Geometry check sheet. Reference: drawing and pictorial views, mm from the part's lowest x, y, z. Coordinates: 2 decimals unless noted, no trailing zeros. Write each loop counter-clockwise with the first axis right and the second up, starting at its lowest first coordinate (ties: lowest second). Pieces come first, ordered by that corner, then holes. Notation, with made-up numbers: (8, 16) -> (52, 16) arc R23 cw to (52, 45) -> close; hole circle Ø9 at (76, 38.25). An arc over 180 degrees is marked (long way). Use a Markdown table: item, result. Add a question column.
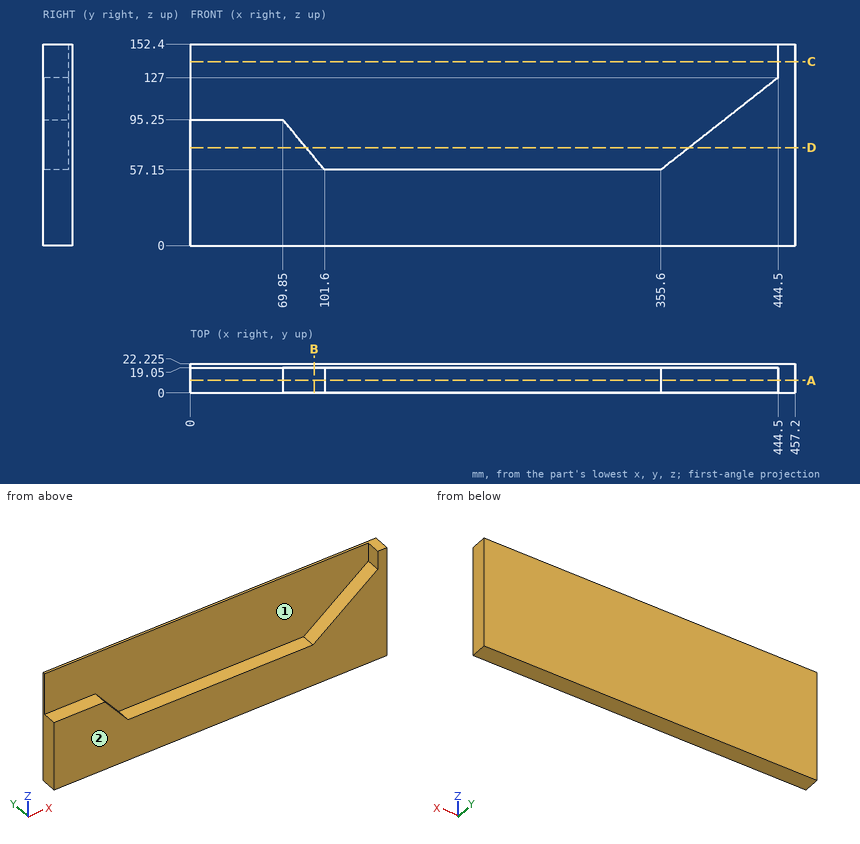
1) Cross-section at B-B on x = 93.5. Record the boundary of the cut face in (y, z) (3 decimals).
2) Cross-section at C-C on z = 139. Record the boundary of the cut face in (x, y) (3 decimals).
3) Gauge pin test, flat ends, axial feed: pin 1 (4 mm diameter, centred on x = 374, y = 13, fed in from +Z); pin 2 (4 mm diameter, centred on x = 322, z = 114.5, fed in from -Y); pin 3 (6 mm diameter, centred on x = 66.5, y = 2.5, fed in from +Z). Record the tip position at first contact, or that the pin passes through.
4) Thickness scan on L1, parallel to Z at x = 284, y = 15.5; L2, parallel to X at y = 11, z = 79; L3, parallel to X at y = 8.25, z = 64. Record the ranges inside material, lowest first.
5) Cross-section at D-D on z = 74. Record the boundary of the cut face in (x, y) (3 decimals), then the cut area to 3 significant figures.
6) Release check for a two-part mould opening along X. For the marked faces 1 and 2 record: released by +X, released by -X, zero draft, split by the parting line, or undercut.
7) Cross-section at A-A on y = 9.5. Record the boundary of the cut face in (x, z), then the cut area to 3 significant figures.
Returned:
| question | item | result |
|---|---|---|
| 1 | outline | (0, 0) -> (22.225, 0) -> (22.225, 152.4) -> (19.05, 152.4) -> (19.05, 66.87) -> (0, 66.87) -> close |
| 2 | outline | (0, 19.05) -> (444.5, 19.05) -> (444.5, 0) -> (457.2, 0) -> (457.2, 22.225) -> (0, 22.225) -> close |
| 3 | pin 1 | stops at z = 73.18 |
| 3 | pin 2 | stops at y = 19.05 |
| 3 | pin 3 | stops at z = 95.25 |
| 4 | L1 | z = 0 to 57.15 |
| 4 | L2 | x = 0 to 83.39, 383.41 to 457.2 |
| 4 | L3 | x = 0 to 95.89, 364.32 to 457.2 |
| 5 | outline | (0, 0) -> (87.558, 0) -> (87.558, 19.05) -> (377.045, 19.05) -> (377.045, 0) -> (457.2, 0) -> (457.2, 22.225) -> (0, 22.225) -> close |
| 5 | area | 4,650 mm² |
| 6 | face 1 | undercut |
| 6 | face 2 | zero draft |
| 7 | outline | (0, 0) -> (457.2, 0) -> (457.2, 152.4) -> (444.5, 152.4) -> (444.5, 127) -> (355.6, 57.15) -> (101.6, 57.15) -> (69.85, 95.25) -> (0, 95.25) -> close |
| 7 | area | 33,700 mm² |
